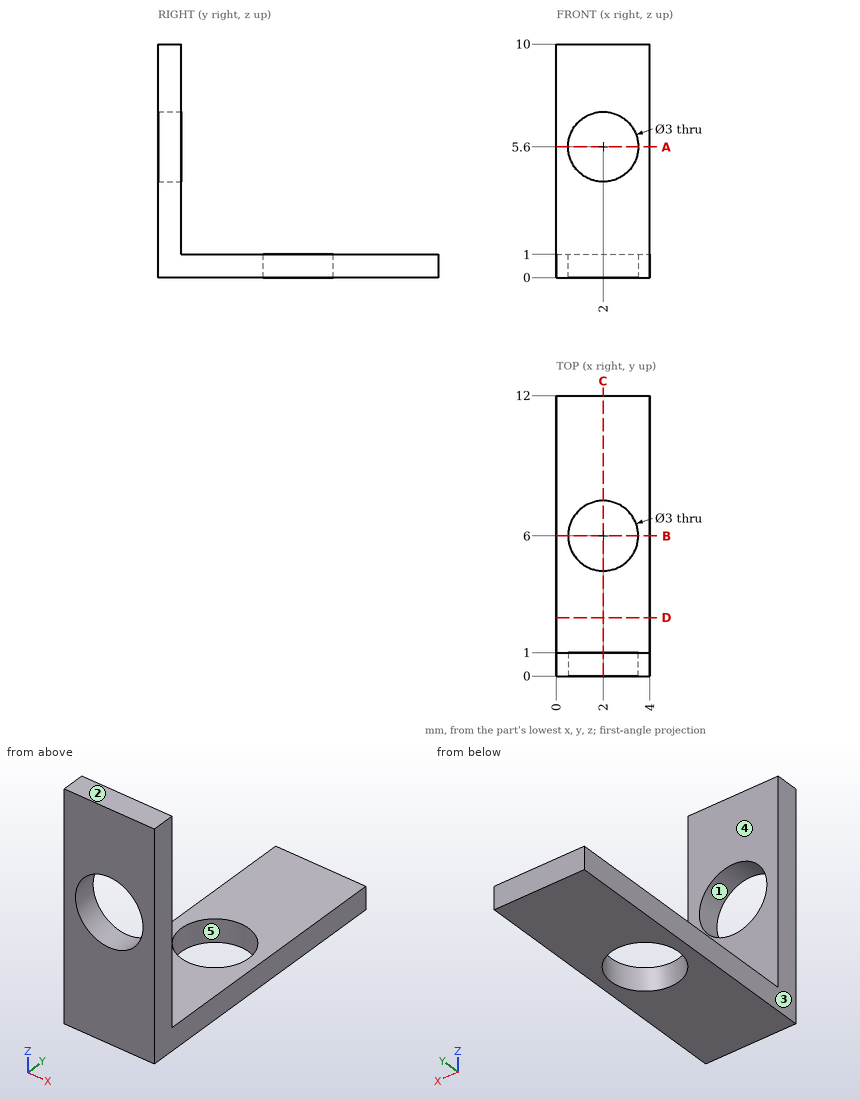
Check sheet for the drawn part. Datum: minimum x, y, z corner. Units: mm. A direction names the side the tool comes from. Round coordinates to 2 decimals unless told otherwise and drop trailing zeros. Order: outer loops, then holes, each group sorted by start corner. A loop starts at its lowest first (then second) coordinate and runs counter-clockwise, first axis right, second up.
(1) Cross-section at C-C, the plane x = 2. Enter the section's corners in (y, z).
(2) Cross-section at D-D, the plane y = 2.5. Enter the section's corners in (x, z).
(3) Cross-section at A-A, the plane z = 5.6. Enter the section's corners in (x, y), and give its area (3 significant figures).
(4) Access from +Z, -Z, +X, -X, +Y, -Y to the whole of each face (thin tool, end or side, straight path). Record for the marked faces 4 and 5.
(5) Go/stop test with flat-tipped pins: P1, Ø1.2, axis at x = 2.5, y = 7.5, coming from the +Z side; P2, Ø1.2, axis at x = 1.5, z = 7, coming from the +Y side. Record where each tip stops, or that it passes through.
(6) Scan lines: probe 1 along Z at (x, y) = (2, 0.8); probe 2 along Y at (x, z) = (2, 0.2); probe 3 along Z at (x, y) = (3.75, 10). Record each from-to range of solid material in increasing order.
(7) Draft check along X on the marked faces 1, 2 and 3. Enter one of: pulls with the +X half, pulls with the -X half, needs draft (parallel to the pull), parting line crosses it, or undercut.
Check sheet entries:
1. outline: (0, 0) - (4.5, 0) - (4.5, 1) - (1, 1) - (1, 4.1) - (0, 4.1) - close; (0, 7.1) - (1, 7.1) - (1, 10) - (0, 10) - close; (7.5, 0) - (12, 0) - (12, 1) - (7.5, 1) - close
2. outline: (0, 0) - (4, 0) - (4, 1) - (0, 1) - close
3. outline: (0, 0) - (0.5, 0) - (0.5, 1) - (0, 1) - close; (3.5, 0) - (4, 0) - (4, 1) - (3.5, 1) - close
3. area: 1.00 mm2
4. face 4: +Z, +X, -X, +Y
4. face 5: +Z, -Z
5. P1: stops at z = 1
5. P2: stops at y = 1
6. probe 1: z = 0 to 4.1, 7.1 to 10
6. probe 2: y = 0 to 4.5, 7.5 to 12
6. probe 3: z = 0 to 1
7. face 1: undercut
7. face 2: needs draft
7. face 3: pulls with the -X half
